CAD build for the part. Positions are in the model's coordinates, mm. A direction names the side the tool comes from. Give positions to 0.01 mm unless a question says otherwise; leave off trailing zeros. Write each loop counter-clockwise with the first axis right and the second up, starting at its lowest first coordinate (ties: lowest second). Pieces come first, ordered by that corner, then holes. Notation, with made-up numbers: (25, -38) -> (70, -38) arc R19 cw to (70, -29) -> close; hole circle Ø2 at (14.5, 15.5). An arc over 180 degrees is marked (long way). Answer as a JSON object with one key per item and string values.
```python
from build123d import *

# Parameters (mm, degrees)
BOSS_EXTRUDE1_DEPTH      = 16
FILLET1_R                = 25
SKETCH2_R                = 7.5
CUT_EXTRUDE1_DEPTH       = 167.901106215
BOSS_EXTRUDE2_DEPTH      = 6
BOSS_EXTRUDE2_DEPTH_BACK = 36
SKETCH3_R                = 25
SKETCH3_R_2              = 14
BOSS_EXTRUDE3_DEPTH      = 16
SKETCH5_R                = 7.5
CUT_EXTRUDE2_DEPTH       = 185.720197269
SKETCH6_W                = 30
SKETCH6_H                = 60
CUT_EXTRUDE3_DEPTH       = 5


with BuildPart() as part:
    # Sketch1 → Boss-Extrude1 (new body)
    with BuildSketch(Plane(origin=(0, 0, 0), x_dir=(1, 0, 0), z_dir=(0, 1, 0))):
        Polygon((0, 0), (142, 0), (142, -70), (0, -90), align=None)
    extrude(amount=BOSS_EXTRUDE1_DEPTH)

    # Fillet1
    fillet1_edges = [part.edges().sort_by_distance(p)[0] for p in [
        (142, 8, 70),
        (0, 8, 90),
    ]]
    fillet(fillet1_edges, radius=FILLET1_R)

    # Sketch2 → Cut-Extrude1 (cut, through all)
    with BuildSketch(Plane(origin=(0, 16, 0), x_dir=(1, 0, 0), z_dir=(0, 1, 0))):
        with Locations(Location((25, -65, 0), (0, 0, 270))):
            Circle(SKETCH2_R)
        with Locations(Location((117, -40, 0), (0, 0, 270))):
            Circle(SKETCH2_R)
    extrude(amount=-CUT_EXTRUDE1_DEPTH, mode=Mode.SUBTRACT)



with BuildPart() as body_2:
    # Sketch3 → Boss-Extrude2 (new, two sides: drawn at the far end of the back side and taken through both)
    with BuildSketch(Plane(origin=(0, 0, 0), x_dir=(-1, 0, 0), z_dir=(0, 0, -1)).offset(-BOSS_EXTRUDE2_DEPTH_BACK)):
        with Locations((-20.64, 70)):
            Circle(SKETCH3_R)
        with Locations((-20.64, 70)):
            Circle(SKETCH3_R_2, mode=Mode.SUBTRACT)
    extrude(amount=BOSS_EXTRUDE2_DEPTH + BOSS_EXTRUDE2_DEPTH_BACK)


with BuildPart() as part_1:
    add(part.part)

    add(body_2.part)  # Boss-Extrude3 merges body 2
    # Sketch4 → Boss-Extrude3 (add)
    with BuildSketch(Plane.XY):
        with BuildLine():
            Line((142, 16), (111.656574903, 45.476470094))
            ThreePointArc((111.656574903, 45.476470094), (106.523670107, 48.826050072), (100.508003955, 50))
            Line((100.508003955, 50), (45.64, 50))
            Line((45.64, 50), (45.64, 70))
            ThreePointArc((45.64, 70), (28.02241153, 46.114858175), (0, 55.893604287))
            Line((0, 55.893604287), (0, 16))
            Line((0, 16), (142, 16))
        make_face()
    extrude(amount=BOSS_EXTRUDE3_DEPTH)

    # Sketch5 → Cut-Extrude2 (cut, through all)
    with BuildSketch(Plane.XY.offset(16)):
        with Locations((97, 36)):
            Circle(SKETCH5_R)
    extrude(amount=-CUT_EXTRUDE2_DEPTH, mode=Mode.SUBTRACT)

    # Sketch6 → Cut-Extrude3 (cut)
    with BuildSketch(Plane.XY.offset(36)):
        with Locations((20.64, 70)):
            Rectangle(SKETCH6_W, SKETCH6_H)
    extrude(amount=-CUT_EXTRUDE3_DEPTH, mode=Mode.SUBTRACT)


solid = part_1.part
```
1) 3-axis set-ups, long thin cutter, end or side, ignore diameter. For faces 1 (the cylindrical face through (136.033, 8.112, 64.483)), 2 (the flat face through (35.64, 70, 34)): which of +Z, -Z, +X, -X, +Y, -Y reach the whole face in a straight line?
Model answer:
{"face 1": "+Z, +X, +Y, -Y", "face 2": "+Z, +Y"}
2) Mould opens along X. For faces 3 (the flat face through (40, 70, 36)), 4 (the cylindrical face through (109.68, 8.11, 38.37)), 5 (the flat face through (45.64, 60, 8)), 6 (the flat face through (0, 10, 23)) say: released by +X, released by -X, zero draft, split by the parting line, or undercut.
Model answer:
{"face 3": "zero draft", "face 4": "undercut", "face 5": "released by +X", "face 6": "released by -X"}
3) Slice it at D-D (z = 40). List the corners of the cut face in (x, y).
Model answer:
{"outline": "(0, 0) -> (109.5, 0) -> (109.5, 16) -> (0, 16) -> close; (124.5, 0) -> (142, 0) -> (142, 16) -> (124.5, 16) -> close"}
4) Slice it at C-C (x = 97). List the corners of the cut face in (y, z).
Model answer:
{"outline": "(0, 0) -> (28.5, 0) -> (28.5, 16) -> (16, 16) -> (16, 76.34) -> (0, 76.34) -> close; (43.5, 0) -> (50, 0) -> (50, 16) -> (43.5, 16) -> close"}
5) Slice it at A-A (z = 24.5). List the corners of the cut face in (x, y).
Model answer:
{"outline": "circle Ø50 at (20.64, 70); (0, 0) -> (142, 0) -> (142, 16) -> (0, 16) -> close; hole circle Ø28 at (20.64, 70)"}
6) Pin check, flat tips, straight feed: pin 1 (12 mm diameter, centred on x = 36.5, z = 57, fed in from +Y); pin 2 (5.5 mm diameter, centred on y = 74, z = 34.5, fed in from +X); pin 3 (8 mm diameter, centred on x = 31.5, y = 29.5, fed in from -Z). Stop position of each tip, or through.
Model answer:
{"pin 1": "stops at y = 16", "pin 2": "stops at x = 45.61", "pin 3": "stops at z = 0"}
7) Wall check: probe 1 along X at (y, z) = (70, 6); probe 2 along Y at (x, z) = (65.5, 20). Give the ranges that are in metal, low to high.
Model answer:
{"probe 1": "x = -4.36 to 6.64, 34.64 to 45.64", "probe 2": "y = 0 to 16"}
8) Slice it at B-B (y = 77). List the corners of the cut face in (x, z), then the cut area to 3 significant figures.
Model answer:
{"outline": "(-3.36, -6) -> (8.52, -6) -> (8.52, 31) -> (5.64, 31) -> (5.64, 36) -> (-3.36, 36) -> close; (32.76, -6) -> (44.64, -6) -> (44.64, 36) -> (35.64, 36) -> (35.64, 31) -> (32.76, 31) -> close", "area": "969 mm2"}
